```python
from build123d import *

# Parameters (mm, degrees)
SM_BASE_FLANGE_1_DEPTH = 40
CUT_EXTRUDE_1_REACH    = 117.721
SKETCH_6_R             = 15
CUT_EXTRUDE_2_DEPTH    = 172.54008278
FILLET_1_R             = 5


# Sheet-metal steps are written as plain solids
with BuildPart() as part:
    # Sketch 1 → 基体-法兰1 (new, symmetric)
    with BuildSketch(Plane(origin=(0, 0, 0), x_dir=(0, 0, -1), z_dir=(1, 0, 0))):
        with BuildLine():
            Line((-70.5, 75), (-70.5, 4))
            ThreePointArc((-70.5, 4), (-69.328427125, 1.171572875), (-66.5, 0))
            Line((-66.5, 0), (66.5, 0))
            ThreePointArc((66.5, 0), (69.328427125, 1.171572875), (70.5, 4))
            Line((70.5, 4), (70.5, 75))
            Line((70.5, 75), (74.5, 75))
            Line((74.5, 75), (74.5, 4))
            ThreePointArc((74.5, 4), (72.156854249, -1.656854249), (66.5, -4))
            Line((66.5, -4), (-66.5, -4))
            ThreePointArc((-66.5, -4), (-72.156854249, -1.656854249), (-74.5, 4))
            Line((-74.5, 4), (-74.5, 75))
            Line((-74.5, 75), (-70.5, 75))
        make_face()
    extrude(amount=SM_BASE_FLANGE_1_DEPTH, both=True)

    # 草图6 → 切除-拉伸1 (cut, up to next)
    with BuildSketch(Plane.XZ.offset(4), mode=Mode.PRIVATE) as cut_extrude_1_sk1:
        with Locations(Location((0, 0, 0), (0, 0, 270))):
            Circle(SKETCH_6_R)
    cut_extrude_1_tool1 = extrude(cut_extrude_1_sk1.sketch, amount=-CUT_EXTRUDE_1_REACH, mode=Mode.PRIVATE) & part.part
    add(cut_extrude_1_tool1.solids().sort_by_distance((0, -4, 0))[0], mode=Mode.SUBTRACT)

    # 草图7 → 切除-拉伸2 (cut, through all)
    with BuildSketch(Plane.XY.offset(74.5)):
        with BuildLine():
            Line((4.5, 57), (4.5, 54))
            ThreePointArc((4.5, 54), (0, 49.5), (-4.5, 54))
            Line((-4.5, 54), (-4.5, 57))
            ThreePointArc((-4.5, 57), (0, 61.5), (4.5, 57))
        make_face()
    extrude(amount=-CUT_EXTRUDE_2_DEPTH, mode=Mode.SUBTRACT)

    # 圆角1
    fillet_1_edges = [part.edges().sort_by_distance(p)[0] for p in [
        (-40, 75, 72.5),
        (-40, 75, -72.5),
        (40, 75, 72.5),
        (40, 75, -72.5),
    ]]
    fillet(fillet_1_edges, radius=FILLET_1_R)


solid = part.part
```
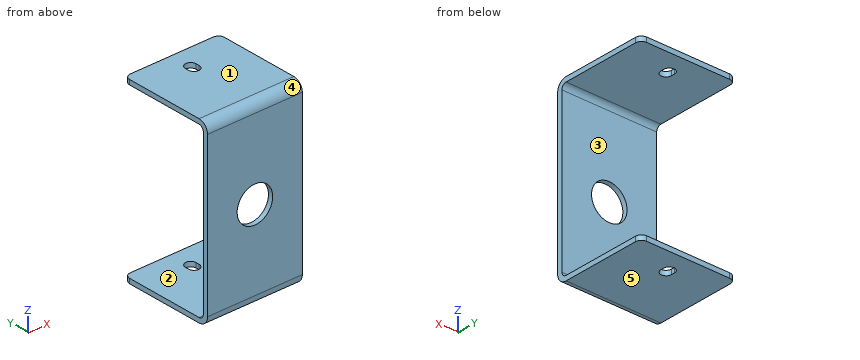
Geometry: final body of the model. Coordinates: model frame, mm. Face numbers are marked on the shaded views. A direction names the side the tool comes from. Round coordinates to 2 decimals unless told otherwise and drop trailing zeros. Write each loop counter-clockwise with the first axis right and the second up, starting at its lowest first coordinate (ties: lowest second). Pieces come first, ordered by that corner, then holes. Notation, with made-up numbers: (83.5, 0.5) -> (119.5, 0.5) arc R11 ccw to (119.5, 20.5) -> close; hole circle Ø6 at (54.5, -20). An arc over 180 degrees is marked (long way). Return JSON: item names as keys, results as strings.
Q1. Ray query, line 1 (Z direction, x = 21, y = 42); line 2 (X direction, y = -2, z = 0); line 3 (Y direction, x = 17.5, z = 66.5). Return the intervals inside material, ascending.
From the geometry:
{"line 1": "-74.5 to -70.5, 70.5 to 74.5", "line 2": "-40 to -15, 15 to 40", "line 3": "-4 to 0"}
Q2. Section D-D on z = 54. Return the cut outline in (x, y), and give its area (3 significant figures).
From the geometry:
{"outline": "(-40, -4) -> (40, -4) -> (40, 0) -> (-40, 0) -> close", "area": "320 mm2"}
Q3. Section C-C on x = 0. Return the cut outline in (y, z), and give its area (3 significant figures).
From the geometry:
{"outline": "(-4, -66.5) arc R8 ccw to (4, -74.5) -> (49.5, -74.5) -> (49.5, -70.5) -> (4, -70.5) arc R4 cw to (0, -66.5) -> (0, -15) -> (-4, -15) -> close; (-4, 15) -> (0, 15) -> (0, 66.5) arc R4 cw to (4, 70.5) -> (49.5, 70.5) -> (49.5, 74.5) -> (4, 74.5) arc R8 ccw to (-4, 66.5) -> close; (61.5, -74.5) -> (75, -74.5) -> (75, -70.5) -> (61.5, -70.5) -> close; (61.5, 70.5) -> (75, 70.5) -> (75, 74.5) -> (61.5, 74.5) -> close", "area": "959 mm2"}
Q4. Set-up query: the marked faces 1 and 2. Return all of +Z, -Z, +X, -X, +Y, -Y with unobstructed straight access to the full face (end or side cutting, diameter ignored); none if empty.
From the geometry:
{"face 1": "+Z, +X, -X, +Y, -Y", "face 2": "+X, -X, +Y"}
Q5. Section B-B on y = 35. Return the cut outline in (x, z).
From the geometry:
{"outline": "(-40, -74.5) -> (40, -74.5) -> (40, -70.5) -> (-40, -70.5) -> close; (-40, 70.5) -> (40, 70.5) -> (40, 74.5) -> (-40, 74.5) -> close"}
Q6. Section A-A on z = -12. Return the cut outline in (x, y).
From the geometry:
{"outline": "(-40, -4) -> (-9, -4) -> (-9, 0) -> (-40, 0) -> close; (9, -4) -> (40, -4) -> (40, 0) -> (9, 0) -> close"}
Q7. Mould query, pull axis Z, two halves, no side actions, for the marked faces 3, 4 and 5. Classes: +Z half, -Z half, draft (parallel to the pull), parting line (faces both ways), or undercut.
From the geometry:
{"face 3": "undercut", "face 4": "+Z half", "face 5": "-Z half"}
